```python
from build123d import *

# Parameters (mm, degrees)
BOSS_EXTRUDE1_DEPTH = 156.2
SKETCH2_R           = 10
SKETCH2_R_2         = 25
CUT_EXTRUDE1_DEPTH  = 26.525992736


with BuildPart() as part:
    # Sketch1 → Boss-Extrude1 (new body)
    with BuildSketch(Plane(origin=(0, 0, 0), x_dir=(1, 0, 0), z_dir=(0, 1, 0))):
        with BuildLine():
            Line((-140, 0), (-140, -20))
            Line((-140, -20), (140, -20))
            Line((140, -20), (140, 0))
            ThreePointArc((140, 0), (0, 5.525992736), (-140, 0))
        make_face()
    extrude(amount=BOSS_EXTRUDE1_DEPTH)

    # Sketch2 → Cut-Extrude1 (cut, through all)
    with BuildSketch(Plane.XY.offset(20)):
        with Locations((-110, 136.2)):
            Circle(SKETCH2_R)
        with Locations((-110, 20)):
            Circle(SKETCH2_R)
        with Locations((110, 20)):
            Circle(SKETCH2_R)
        with Locations((110, 136.2)):
            Circle(SKETCH2_R)
        with Locations((0, 78.1)):
            Circle(SKETCH2_R_2)
    extrude(amount=-CUT_EXTRUDE1_DEPTH, mode=Mode.SUBTRACT)


solid = part.part
```
The listing builds one solid part. Answer for the finished solid, in the listing's coordinates (mm). Give positions to 0.01 mm unless a question says otherwise; leave off trailing zeros. Write each loop counter-clockwise with the first axis right and the second up, starting at its lowest first coordinate (ties: lowest second). Pieces come first, ordered by that corner, then holes. Notation, with made-up numbers: (70, 48.25) - (119, 48.25) arc R12 ccw to (119, 60.25) - close; hole circle Ø7 at (44.25, 55.5). An arc over 180 degrees is marked (long way). Use one line per item in the form item = value. Start each with the question number.
1) The mould has two halves that part along X. Classify faces 1 (the face through (33.104, 77.007, -5.217)), 2 (the face through (-2, 0, 7)), 3 (the face through (-3.255, 102.887, 7.416)): pulls with the +X half, pulls with the -X half, needs draft (parallel to the pull), parting line crosses it, or undercut.
2) Flat-ended cylindrical pins translate along their axes: pin 1 Ø1 at (x, z) = (-44.5, 1.5) entering from -Y; pin 2 Ø23 at (x, y) = (110, 136.2) entering from -Z. Find the tip coordinate at first contact, or state that the pin passes through.
3) Find section B-B on y = 78.1. Determine the outline of the cut face in (x, z).
4) Find section A-A on x = 0. Determine the outline of the cut face in (y, z), plus the area to 3 significant figures.
5) Find section C-C on z = 9. Determine the outline of the cut face in (x, y), plus the area to 3 significant figures.
6) Find section D-D on x = -110. Determine the outline of the cut face in (y, z), plus the area to 3 significant figures.
7) Consider line 1 along Y through (x, z) = (-110, 3.25); line 2 along Y through (x, z) = (106, -0.5); line 3 along Y through (x, z) = (0, 7). Determine where each line is inside the solid, lowest interval first. Write a range as from..to.
Geometry results:
q1.face_1 = parting line crosses it
q1.face_2 = needs draft
q1.face_3 = undercut
q2.pin_1 = 0
q2.pin_2 = -2.79
q3.outline = (-140, 0) arc R1776.2 ccw to (-25, -5.35) - (-25, 20) - (-140, 20) - close; (25, -5.35) arc R1776.2 ccw to (140, 0) - (140, 20) - (25, 20) - close
q4.outline = (0, -5.53) - (53.1, -5.53) - (53.1, 20) - (0, 20) - close; (103.1, -5.53) - (156.2, -5.53) - (156.2, 20) - (103.1, 20) - close
q4.area = 2,710 mm2
q5.outline = (-140, 0) - (140, 0) - (140, 156.2) - (-140, 156.2) - close; hole circle Ø20 at (-110, 20); hole circle Ø20 at (-110, 136.2); hole circle Ø50 at (0, 78.1); hole circle Ø20 at (110, 20); hole circle Ø20 at (110, 136.2)
q5.area = 40,500 mm2
q6.outline = (0, -2.12) - (10, -2.12) - (10, 20) - (0, 20) - close; (30, -2.12) - (126.2, -2.12) - (126.2, 20) - (30, 20) - close; (146.2, -2.12) - (156.2, -2.12) - (156.2, 20) - (146.2, 20) - close
q6.area = 2,570 mm2
q7.line_1 = 0..10, 30..126.2, 146.2..156.2
q7.line_2 = 0..10.83, 29.17..127.03, 145.37..156.2
q7.line_3 = 0..53.1, 103.1..156.2
